from build123d import *

# Parameters (mm, degrees)
SKETCH1_W           = 178
SKETCH1_H           = 85
SKETCH1_R           = 2.6
BOSS_EXTRUDE1_DEPTH = 10
M8_TAPPED_HOLE1_D   = 6.8


with BuildPart() as part:
    # Sketch1 → Boss-Extrude1 (new body)
    with BuildSketch(Plane.XY):
        Rectangle(SKETCH1_W, SKETCH1_H)
        with Locations((-77, -30)):
            Circle(SKETCH1_R, mode=Mode.SUBTRACT)
        with Locations((-41, -30)):
            Circle(SKETCH1_R, mode=Mode.SUBTRACT)
        with Locations((-41, 30)):
            Circle(SKETCH1_R, mode=Mode.SUBTRACT)
        with Locations((-77, 30)):
            Circle(SKETCH1_R, mode=Mode.SUBTRACT)
        with Locations((-17.5, -18.5)):
            Circle(SKETCH1_R, mode=Mode.SUBTRACT)
        with Locations((17.5, -18.5)):
            Circle(SKETCH1_R, mode=Mode.SUBTRACT)
        with Locations((17.5, 5.5)):
            Circle(SKETCH1_R, mode=Mode.SUBTRACT)
        with Locations((-17.5, 5.5)):
            Circle(SKETCH1_R, mode=Mode.SUBTRACT)
        with Locations((77, -30)):
            Circle(SKETCH1_R, mode=Mode.SUBTRACT)
        with Locations((41, -30)):
            Circle(SKETCH1_R, mode=Mode.SUBTRACT)
        with Locations((41, 30)):
            Circle(SKETCH1_R, mode=Mode.SUBTRACT)
        with Locations((77, 30)):
            Circle(SKETCH1_R, mode=Mode.SUBTRACT)
    extrude(amount=BOSS_EXTRUDE1_DEPTH)

    # M8 Tapped Hole1 (through all)
    with Locations(Plane.XY.offset(10)):
        with Locations((59, 30.5), (-59, 30.5), (-59, -30.5), (59, -32)):
            Hole(M8_TAPPED_HOLE1_D / 2)


solid = part.part
The model under review builds one solid part; all positions refer to its coordinate system, in mm. Round coordinates to 2 decimals unless told otherwise and drop trailing zeros. Write each loop counter-clockwise with the first axis right and the second up, starting at its lowest first coordinate (ties: lowest second). Pieces come first, ordered by that corner, then holes. Notation, with made-up numbers: M 71,39 L 104,39 A37 ccw 104,75 Z; hole C 22.5,29 d7. An arc over 180 degrees is marked long. Answer as CSV lines item,"result". Start each with the question number.
Q1. The part is to be moulded in two halves that separate along X. For faces 1 (the face through (-15.02, -17.72, 4.93)), 2 (the face through (-1, 42.5, 5)), 3 (the face through (-15.02, 6.28, 4.93)), 4 (the face through (-89, -1, 5)), say which applies: +X half, -X half, draft (parallel to the pull), parting line (faces both ways), or undercut.
Q2. Consider section B-B, the plane x = 59. Give the boundary of the cut face in (y, z), then the cut area to 3 significant figures.
Q3. Wall thickness on line 1 along Y through (x, z) = (-17.5, 2.5); line 2 along Y through (x, z) = (-56, 7); line 3 along X through (y, z) = (-18, 3.75): over which ranges is each line inside the solid? List them lowest first.
Q4. Consider section C-C, the plane z = 6.5. State how many separate pieces and enclosed holes the cut face has, then the cut area to 3 significant figures.
Q5. Consider section A-A, the plane y = 5.5. Give the boundary of the cut face in (x, z), then the cut area to 3 significant figures.
Result set:
1,face 1,"undercut"
1,face 2,"draft"
1,face 3,"undercut"
1,face 4,"-X half"
2,outline,"M -42.5,0 L -35.4,0 L -35.4,10 L -42.5,10 Z; M -28.6,0 L 27.1,0 L 27.1,10 L -28.6,10 Z; M 33.9,0 L 42.5,0 L 42.5,10 L 33.9,10 Z"
2,area,"714 mm²"
3,line 1,"y = -42.5 to -21.1, -15.9 to 2.9, 8.1 to 42.5"
3,line 2,"y = -42.5 to -32.1, -28.9 to 28.9, 32.1 to 42.5"
3,line 3,"x = -89 to -20.05, -14.95 to 14.95, 20.05 to 89"
4,separate pieces,"1"
4,enclosed holes,"16"
4,area,"14,700 mm²"
5,outline,"M -89,0 L -20.1,0 L -20.1,10 L -89,10 Z; M -14.9,0 L 14.9,0 L 14.9,10 L -14.9,10 Z; M 20.1,0 L 89,0 L 89,10 L 20.1,10 Z"
5,area,"1,680 mm²"
